from build123d import *

# Parameters (mm, degrees)
BOSS_EXTRUDE1_DEPTH      = 71.4375
BOSS_EXTRUDE1_DEPTH_BACK = 71.4375
F_10_CLEARANCE_HOLE1_D   = 5.1054
F_10_CLEARANCE_HOLE2_D   = 5.1054


with BuildPart() as part:
    # Sketch3 → Boss-Extrude1 (new, two sides: drawn at the far end of the back side and taken through both)
    with BuildSketch(Plane.XY.offset(-BOSS_EXTRUDE1_DEPTH_BACK)):
        Polygon((23.8125, -9.525), (23.8125, -12.7), (-1.5875, -12.7), (-1.5875, 9.525), (-23.8125, 9.525), (-23.8125, 12.7), (1.5875, 12.7), (1.5875, -9.525), align=None)
    extrude(amount=BOSS_EXTRUDE1_DEPTH + BOSS_EXTRUDE1_DEPTH_BACK)

    # #10 Clearance Hole1 (through all)
    with Locations(Plane(origin=(0, 12.7, 0), x_dir=(1, 0, 0), z_dir=(0, 1, 0))):
        with Locations((-14.2875, -50.799999492), (-14.2875, 50.800000508)):
            Hole(F_10_CLEARANCE_HOLE1_D / 2)

    # #10 Clearance Hole2 (through all)
    with Locations(Plane(origin=(0, -9.525, 0), x_dir=(1, 0, 0), z_dir=(0, 1, 0))):
        with Locations((8.89, -50.799999492), (8.89, 50.799700006)):
            Hole(F_10_CLEARANCE_HOLE2_D / 2)


solid = part.part
Can you work these out from the model? Positions are in its coordinate system, mm. A direction names the side the tool comes from. Coordinates: 2 decimals unless noted, no trailing zeros. Order: outer loops, then holes, each group sorted by start corner. A loop starts at its lowest first (then second) coordinate and runs counter-clockwise, first axis right, second up. Notation, with made-up numbers: (85, 55.25) - (92, 55.25) arc R23 ccw to (92, 75.25) - close; hole circle Ø5 at (-36, 86.5). An arc over 180 degrees is marked (long way). Answer as a JSON object with one key per item and string values. Group by question number.
Q1. On a 3-axis mill with a long thin cutter (end or side, diameter ignored), from which of +Z, -Z, +X, -X, +Y, -Y can I reach the whole of each face in a straight line? I mean faces 4 (the face through (13, -9.525, -1)), 5 (the face through (-11, 12.7, -1)), 6 (the face through (-13, 9.525, -1)). Say none if no direction works.
Q2. Will these pins go through, and if not, where does the flat tip stop? P1, Ø2, axis at x = 5.5, z = -4.5, coming from the +Y side (3 decimals); P2, Ø1.5, axis at y = -4.5, z = -18, coming from the +X side; P3, Ø12, axis at x = 15, y = 0.5, coming from the -Z side; P4, Ø12, axis at x = 14, y = -8, coming from the -Z side.
Q3. We'd pull the mould along X, two halves only. Please class faces 1 (the face through (9.4, -11.1, -48.3)), 2 (the face through (11, -12.7, -1)), 3 (the face through (-1.588, -2, -1)): +X half, -X half, draft (parallel to the pull), parting line (faces both ways), or undercut.
Q4. I need wall thicknesses on line 1 (Z direction, x = 8.89, y = -10.8); line 2 (X direction, y = 10.9, z = 50.8); line 3 (X direction, y = -11.05, z = 50.8). Which ranges of each line are inside material? Lowest first, please. Write a range as from..to.
Q5. Imagine slicing it at D-D (z = 7.5). Please give me the cut outline in (x, y) (1 decimal).
Q6. Imagine slicing it at C-C (y = 10.75). Please give me the cut outline in (x, z).
Q7. Imagine slicing it at B-B (x = 8.89). Please give me the cut outline in (y, z) (1 decimal).
Q8. Imagine slicing it at A-A (z = 50.8). Please give me the cut outline in (x, y) (1 decimal), and give its area (3 significant figures).
Determined:
{
 "1": {"face 4": "+Z, -Z, +X, +Y", "face 5": "+Z, -Z, +X, -X, +Y", "face 6": "+Z, -Z, -X, -Y"},
 "2": {"P1": "stops at y = -9.525", "P2": "stops at x = 1.59", "P3": "passes through", "P4": "stops at z = -71.44"},
 "3": {"face 1": "undercut", "face 2": "draft", "face 3": "-X half"},
 "4": {"line 1": "z = -71.44..-53.35, -48.25..48.25, 53.35..71.44", "line 2": "x = -23.81..-16.84, -11.73..1.59", "line 3": "x = -1.59..6.34, 11.44..23.81"},
 "5": {"outline": "(-23.8, 9.5) - (-1.6, 9.5) - (-1.6, -12.7) - (23.8, -12.7) - (23.8, -9.5) - (1.6, -9.5) - (1.6, 12.7) - (-23.8, 12.7) - close"},
 "6": {"outline": "(-23.81, -71.44) - (1.59, -71.44) - (1.59, 71.44) - (-23.81, 71.44) - close; hole circle Ø5.11 at (-14.29, -50.8); hole circle Ø5.11 at (-14.29, 50.8)"},
 "7": {"outline": "(-12.7, -71.4) - (-9.5, -71.4) - (-9.5, -53.4) - (-12.7, -53.4) - close; (-12.7, -48.2) - (-9.5, -48.2) - (-9.5, 48.2) - (-12.7, 48.2) - close; (-12.7, 53.4) - (-9.5, 53.4) - (-9.5, 71.4) - (-12.7, 71.4) - close"},
 "8": {"outline": "(-23.8, 9.5) - (-16.8, 9.5) - (-16.8, 12.7) - (-23.8, 12.7) - close; (-11.7, 9.5) - (-1.6, 9.5) - (-1.6, -12.7) - (6.3, -12.7) - (6.3, -9.5) - (1.6, -9.5) - (1.6, 12.7) - (-11.7, 12.7) - close; (11.4, -12.7) - (23.8, -12.7) - (23.8, -9.5) - (11.4, -9.5) - close", "area": "189 mm2"}
}
